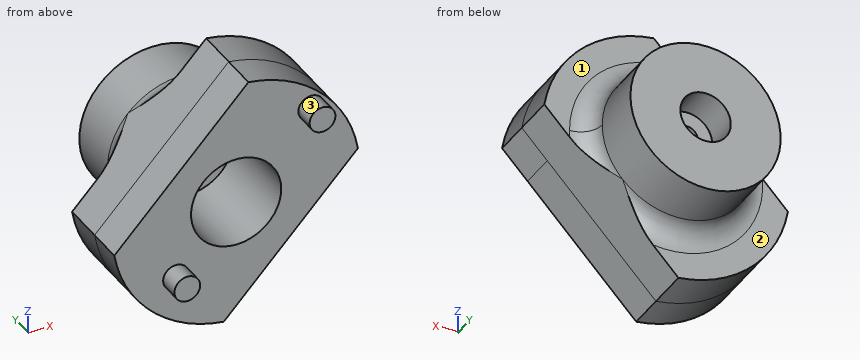
Autodesk Inventor part; units mm, degrees
ref_plane "YZ Plane" through (0, 0, 0) normal (1, 0, 0) x (0, 1, 0)
ref_plane "XZ Plane" through (0, 0, 0) normal (0, 1, 0) x (-1, 0, 0)
ref_plane "XY Plane" through (0, 0, 0) normal (0, 0, 1) x (1, 0, 0)
sketch "Skizze1" plane through (0, 0, 0) normal (0, 1, 0) x (-1, 0, 0)
  circle A0 centre (0, 0) radius 15
  dimension "d0" = 30
extrude "Extrusion1" add sketch "Skizze1" along normal blind 14
sketch "Skizze2" plane through (0, 0, 0) normal (0, -1, 0) x (1, 0, 0)
  line L0 (14.3188, 0.9) -> (12.9688, 0.9)
  line L1 (12.9688, -0.9) -> (14.3188, -0.9)
  line L2 (14.3188, -0.9) -> (14.3188, 0.9)
  line L3 (-21.3175, 0) -> (21.3175, 0)
  arc A0 (12.9688, 0.9) -> (0.9, 12.9688) centre (0, 0) ccw
  line L4 (-0.9, -12.9688) -> (-0.9, -14.3188)
  line L5 (-0.9, -14.3188) -> (0.9, -14.3188)
  line L6 (0.9, -14.3188) -> (0.9, -12.9688)
  line L7 (-12.9688, 0.9) -> (-14.3188, 0.9)
  line L8 (-14.3188, 0.9) -> (-14.3188, -0.9)
  line L9 (-14.3188, -0.9) -> (-12.9688, -0.9)
  line L10 (-0.9, 12.9688) -> (-0.9, 14.3188)
  line L11 (-0.9, 14.3188) -> (0.9, 14.3188)
  line L12 (0.9, 14.3188) -> (0.9, 12.9688)
  line L13 (0, -21.3175) -> (0, 21.3175)
  line L14 (-21.3175, 0) -> (21.3175, 0)
  arc A1 (0.9, -12.9688) -> (12.9688, -0.9) centre (0, 0) ccw
  arc A2 (-12.9688, -0.9) -> (-0.9, -12.9688) centre (0, 0) ccw
  arc A3 (-0.9, 12.9688) -> (-12.9688, 0.9) centre (0, 0) ccw
  circle A4 centre (0, 0) radius 4.2
  circle A5 centre (7, 7.1414) radius 1.2
  circle A6 centre (-5.6, -5.7131) radius 1.2
  dimension "d4" = 0.9
  dimension "d5" = 0.9
  dimension "d8" = 1.35
  dimension "d9" = 1.35
  dimension "d10" = 1.8
  dimension "d11" = 0.9
  dimension "d12" = 1.35
  dimension "d13" = 1.8
  dimension "d14" = 0.9
  dimension "d15" = 0.9
  dimension "d16" = 1.35
  dimension "d17" = 8.4
  dimension "d18" = 2.4
  dimension "d19" = 2.4
  dimension "d20" = 8
  dimension "d21" = 10
  dimension "d22" = 7
  dimension "d23" = 5.6
  dimension "d50" = 13
  dimension "d51" = 13
  dimension "d52" = 1.35
  dimension "d53" = 1.35
  dimension "d54" = 1.35
extrude "Extrusion2" cut sketch "Skizze2" against normal blind 3 contours L2 L3 A4 L13 L11 L12 A0 L0 | L2 L1 A1 L6 L5 L13 A4 L3 | A4 L3 L8 L7 A3 L10 L11 L13 | L13 L5 L4 A2 L9 L8 L3 A4
sketch "Skizze4" plane through (7, 0, 7.1414) normal (0, -1, 0) x (1, 0, 0)
  circle A0 centre (-7, -7.1414) radius 4.2
  circle A1 centre (-12.6, -12.8546) radius 1.2
  circle A2 centre (0, 0) radius 1.2
  line L0 (-7, -28.1414) -> (-7, 13.8586)
  dimension "d26" = 2.4
  dimension "d27" = 5.6
  dimension "d28" = 8
  dimension "d44" = 8.4
  dimension "d45" = 2.4
extrude "Extrusion3" add sketch "Skizze4" along normal blind 2
sketch "Skizze5" plane through (0, 14, 0) normal (0, 1, 0) x (1, 0, 0)
  circle A0 centre (0, 0) radius 19.262
  circle A1 centre (0, 0) radius 7
  dimension "d31" = 14
extrude "Extrusion4" cut sketch "Skizze5" against normal blind 7
fillet "Rundung1" radius 1 8 edges at (12.9688, 1.5, -0.9) (12.9688, 1.5, 0.9) (0.9, 1.5, -12.9688) (-0.9, 1.5, -12.9688) (-12.9688, 1.5, -0.9) (-12.9688, 1.5, 0.9) (-0.9, 1.5, 12.9688) (0.9, 1.5, 12.9688)
sketch "Skizze8" plane through (0, 14, 0) normal (0, 1, 0) x (1, 0, 0)
  circle A0 centre (0, 0) radius 1
  dimension "d46" = 2
extrude "Extrusion7" cut sketch "Skizze8" against normal blind 7
fillet "Rundung2" radius 2 1 edges at (-7, 7, 0)
sketch "Skizze9" plane through (0, -2, 0) normal (0, -1, 0) x (1, 0, 0)
  line L0 (18.2687, 9.2162) -> (-7.478, -18.1772)
  line L1 (-7.478, -18.1772) -> (18.2687, -18.1772)
  line L2 (18.2687, -18.1772) -> (18.2687, 9.2162)
  line L3 (8.0673, 18.8043) -> (-17.6793, -8.5891)
  line L4 (-17.6793, -8.5891) -> (-17.6793, 18.8043)
  line L5 (-17.6793, 18.8043) -> (8.0673, 18.8043)
  point P0 (0, 0)
  dimension "d55" = 7
  dimension "d56" = 7
extrude "Extrusion8" cut sketch "Skizze9" against normal blind 50
sketch "Skizze10" plane through (0, -2, 0) normal (0, -1, 0) x (1, 0, 0)
  circle A0 centre (0, 0) radius 11.5
  circle A1 centre (0, 0) radius 18.9246
  dimension "d61" = 23
extrude "Extrusion9" cut sketch "Skizze10" against normal blind 10
sketch "Skizze11" plane through (0, -2, 0) normal (0, -1, 0) x (1, 0, 0)
  circle A0 centre (0, 0) radius 1
  circle A1 centre (0, 0) radius 4.2
extrude "Extrusion10" cut sketch "Skizze11" against normal blind 10 contours A0 | A1
sketch "Skizze13" plane through (0, 3, 0) normal (0, -1, 0) x (1, 0, 0)
  circle A0 centre (7, 7.1414) radius 1.2
  circle A1 centre (7, 7.1414) radius 1.2
  circle A2 centre (-5.6, -5.7131) radius 1.2
  circle A3 centre (-5.6, -5.7131) radius 1.2
  arc A4 (11.3495, 1.8544) -> (1.1481, 11.4425) centre (0, 0) ccw
  line L0 (11.3495, 1.8544) -> (8.9749, -0.6721)
  line L1 (11.3495, 1.8544) -> (-1.1481, -11.4425)
  line L2 (1.1481, 11.4425) -> (-11.3495, -1.8544)
  line L3 (1.2265, -8.916) -> (-1.1481, -11.4425)
  arc A5 (-11.3495, -1.8544) -> (-1.1481, -11.4425) centre (0, 0) ccw
  circle A6 centre (0, 0) radius 4.2
extrude "Extrusion11" add sketch "Skizze13" along normal blind 3.5
sketch "Skizze14" plane through (7, -2, 7.1414) normal (0, -1, 0) x (1, 0, 0)
  circle A0 centre (0, 0) radius 1.2
  circle A1 centre (0, 0) radius 1.2
  circle A2 centre (-12.6, -12.8546) radius 1.2
  circle A3 centre (-12.6, -12.8546) radius 1.2
  point P0 (-7, -7.1414)
extrude "Extrusion12" add sketch "Skizze14" along normal blind 0.5
sketch "Skizze15" plane through (0, 14, 0) normal (0, 1, 0) x (1, 0, 0)
  circle A0 centre (0, 0) radius 1
  circle A1 centre (0, 0) radius 2.35
  dimension "d68" = 4.7
extrude "Extrusion13" cut sketch "Skizze15" against normal blind 3.3 contours A0 | A1
properties part number "Adaptation_on_OPdevside_4_1"
For this review, take the finished solid that the model builds, in its own axes (mm). Face numbers are marked on the shaded views. A direction names the side the tool comes from. Coordinates: 2 decimals unless noted, no trailing zeros. Loops run counter-clockwise (first coordinate to the right, second up) from the corner with the lowest first, then second, coordinate; pieces in that order, holes last.
1. For the marked faces 1, 2 and 3, list the 3-axis set-ups (+Z, -Z, +X, -X, +Y, -Y) from which the entire face can be reached by the end or side of a thin tool; tool diameter is ignored.
2. Add section B-B, the plane y = 0.25. Give the boundary of the cut face in (x, z).
3. Add section A-A, the plane x = 0. Give the boundary of the cut face in (y, z).
4. For line 1 (X direction, y = 9.95, z = 0); line 2 (X direction, y = 13.25, z = 0), list the stretches that pass through material, from the lowest coordinate up.
5. Insertion check: P1, Ø6, axis at x = -3, z = -7, coming from the +Y side; P2, Ø8, axis at x = -5.5, y = 9, coming from the +Z side; P3, Ø9.5, axis at x = 0, z = 0, coming from the -Y side; P4, Ø3, axis at y = 6, z = 4, coming from the +X side (3 decimals). Each pin has a flat end and moves straight along its axis. Give the tip position at first contact, or say it passes through.
Result:
1. face 1: +Z, +X, +Y
1. face 2: -Z, -X, +Y
1. face 3: -Y
2. outline: (-11.35, -1.85) arc R11.5 ccw to (-1.15, -11.44) - (8.97, -0.67) - (11.35, 1.85) arc R11.5 ccw to (1.15, 11.44) - close; hole circle Ø8.4 at (0, 0)
3. outline: (-0.5, -10.22) - (7, -10.22) - (7, -9) arc R2 cw to (9, -7) - (14, -7) - (14, -2.35) - (10.7, -2.35) - (10.7, -1) - (8, -1) - (8, -4.2) - (-0.5, -4.2) - close; (-0.5, 4.2) - (8, 4.2) - (8, 1) - (10.7, 1) - (10.7, 2.35) - (14, 2.35) - (14, 7) - (9, 7) arc R2 cw to (7, 9) - (7, 10.22) - (-0.5, 10.22) - close
4. line 1: x = -7 to -1, 1 to 7
4. line 2: x = -7 to -2.35, 2.35 to 7
5. P1: stops at y = 14
5. P2: stops at z = 8.12
5. P3: stops at y = -0.5
5. P4: stops at x = 11.225
